```python
from build123d import *

# Parameters (mm, degrees)
BOSS_EXTRUDE1_DEPTH = 49
FILLET1_R           = 5
SKETCH2_R           = 7.25
BOSS_EXTRUDE2_DEPTH = 25
CUT_EXTRUDE1_START  = -15
CUT_EXTRUDE1_DEPTH  = 15


with BuildPart() as part:
    # Sketch1 → Boss-Extrude1 (new body)
    with BuildSketch(Plane.XY):
        with BuildLine():
            Line((-6.562511766, 6.562511766), (-1.975851033, 35.809859155))
            ThreePointArc((-1.975851033, 35.809859155), (0, 37.5), (1.975851033, 35.809859155))
            Line((1.975851033, 35.809859155), (6.562511766, 6.562511766))
            Line((6.562511766, 6.562511766), (35.809859155, 1.975851033))
            ThreePointArc((35.809859155, 1.975851033), (37.5, 0), (35.809859155, -1.975851033))
            Line((35.809859155, -1.975851033), (6.562511766, -6.562511766))
            Line((6.562511766, -6.562511766), (1.975851033, -35.809859155))
            ThreePointArc((1.975851033, -35.809859155), (0, -37.5), (-1.975851033, -35.809859155))
            Line((-1.975851033, -35.809859155), (-6.562511766, -6.562511766))
            Line((-6.562511766, -6.562511766), (-35.809859155, -1.975851033))
            ThreePointArc((-35.809859155, -1.975851033), (-37.5, 0), (-35.809859155, 1.975851033))
            Line((-35.809859155, 1.975851033), (-6.562511766, 6.562511766))
        make_face()
    extrude(amount=BOSS_EXTRUDE1_DEPTH)

    # Fillet1
    fillet1_edges = [part.edges().sort_by_distance(p)[0] for p in [
        (-6.562511766, 6.562511766, 24.5),
        (6.562511766, 6.562511766, 24.5),
        (6.562511766, -6.562511766, 24.5),
        (-6.562511766, -6.562511766, 24.5),
    ]]
    fillet(fillet1_edges, radius=FILLET1_R)

    # Sketch2 → Boss-Extrude2 (add)
    with BuildSketch(Plane(origin=(0, 0, 0), x_dir=(-1, 0, 0), z_dir=(0, 0, -1))):
        with Locations(Location((0, 0, 0), (0, 0, 180))):
            Circle(SKETCH2_R)
    extrude(amount=BOSS_EXTRUDE2_DEPTH)

    # Sketch3 → Cut-Extrude1 (cut)
    with BuildSketch(Plane(origin=(0, 0, -25), x_dir=(-1, 0, 0), z_dir=(0, 0, -1)).offset(CUT_EXTRUDE1_START)):
        with BuildLine():
            Line((6.968679932, -2), (-6.968679932, -2))
            ThreePointArc((-6.968679932, -2), (0, -7.25), (6.968679932, -2))
        make_face()
    extrude(amount=CUT_EXTRUDE1_DEPTH, mode=Mode.SUBTRACT)


solid = part.part
```
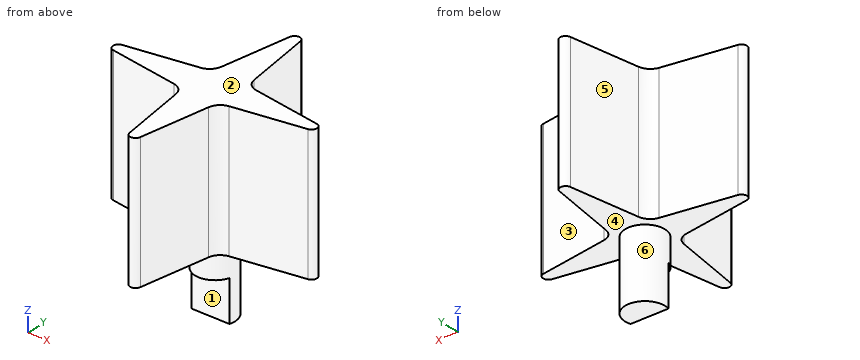
Work out the finished part from the listing and answer in its coordinate system (mm). Face numbers are marked on the shaded views. A direction names the side the tool comes from. Coordinates: 2 decimals unless noted, no trailing zeros. Loops run counter-clockwise (first coordinate to the right, second up) from the corner with the lowest first, then second, coordinate; pieces in that order, holes last.
1) Flat-ended cylindrical pins translate along their axes: pin 1 (6 mm diameter, centred on x = -18, z = 30.5, fed in from +Y); pin 2 (4 mm diameter, centred on x = 1.5, y = -4.5, fed in from -Z); pin 3 (1 mm diameter, centred on y = -21, z = 12.5, fed in from +X). Find the tip coordinate at first contact, or state that the pin passes through.
Results:
pin 1: stops at y = 5.24
pin 2: stops at z = -10
pin 3: stops at x = 4.38
2) Section C-C (z = 30) is taken. Give the vertices of the cut face in (x, y).
Results:
outline: (-35.81, -1.98) - (-10.16, -6) arc R5 cw to (-6, -10.16) - (-1.98, -35.81) arc R2 ccw to (1.98, -35.81) - (6, -10.16) arc R5 cw to (10.16, -6) - (35.81, -1.98) arc R2 ccw to (35.81, 1.98) - (10.16, 6) arc R5 cw to (6, 10.16) - (1.98, 35.81) arc R2 ccw to (-1.98, 35.81) - (-6, 10.16) arc R5 cw to (-10.16, 6) - (-35.81, 1.98) arc R2 ccw to start
3) Section B-B (x = 0) is taken. Give the vertices of the cut face in (y, z).
Results:
outline: (-37.5, 0) - (-7.25, 0) - (-7.25, -10) - (-2, -10) - (-2, -25) - (7.25, -25) - (7.25, 0) - (37.5, 0) - (37.5, 49) - (-37.5, 49) - close
4) Section A-A (y = 0) is taken. Give the vertices of the cut face in (x, z).
Results:
outline: (-37.5, 0) - (-7.25, 0) - (-7.25, -25) - (7.25, -25) - (7.25, 0) - (37.5, 0) - (37.5, 49) - (-37.5, 49) - close
5) For the marked faces 1 and 2, determine the directions among +Z, -Z, +X, -X, +Y, -Y from which every point of the face is accessible in a straight line to the end or side of a thin tool.
Results:
face 1: -Z, +X, -X, -Y
face 2: +Z, +X, -X, +Y, -Y
6) For a pull along X with two mould halves and no side action, classify the marked faces 3, 4, 5 and 6 as +X half, -X half, draft (parallel to the pull), parting line (faces both ways), or undercut.
Results:
face 3: +X half
face 4: draft
face 5: -X half
face 6: parting line
7) Consider probe 1 along Y at (x, z) = (2, -16.5); probe 2 along Z at (x, y) = (-1, -11); probe 3 along Z at (x, y) = (-4, -4). Determine where each line is inside the solid, lowest interval first.
Results:
probe 1: y = -2 to 6.97
probe 2: z = 0 to 49
probe 3: z = -10 to 49
8) Section D-D (z = -19) is taken. Give the vertices of the cut face in (x, y).
Results:
outline: (-6.97, -2) - (6.97, -2) arc R7.25 ccw (long way) to start
